from build123d import *

# Parameters (mm, degrees)
F0_W     = 2
F0_H     = 10
F1_DEPTH = 2
F3_D     = 1
F3_DEPTH = 8
F5_D     = 1
F5_DEPTH = 8


with BuildPart() as f1:
    # F0 (on Front) → F1 (new body)
    with BuildSketch(Plane.XZ):
        Rectangle(F0_W, F0_H)
    extrude(amount=F1_DEPTH)

    # F3
    with Locations(Plane.XZ.offset(2)):
        with Locations((0, 4)):
            Hole(F3_D / 2, depth=F3_DEPTH)

    # F5
    with Locations(Plane.YZ.offset(1)):
        with Locations((-1, 2.5)):
            Hole(F5_D / 2, depth=F5_DEPTH)


solid = f1.part
The model under review builds one solid part; all positions refer to its coordinate system, in mm. Round coordinates to 2 decimals unless told otherwise and drop trailing zeros. Loops run counter-clockwise (first coordinate to the right, second up) from the corner with the lowest first, then second, coordinate; pieces in that order, holes last. Notation, with made-up numbers: (-7, -33.75) -> (37, -33.75) arc R17 cw to (37, -3.75) -> close; hole circle Ø5 at (-7.5, -12.75). An arc over 180 degrees is marked (long way). Return JSON: item names as keys, results as strings.
(1) The part is to be moulded in two halves that separate along Y. For faces 1 (the cylindrical face through (0, -1, 3)), 2 (the flat face through (0, -1, -5)), 3 (the flat face through (0, -2, 0)), say which applies: released by +Y, released by -Y, zero draft, split by the parting line, or undercut.
Solved:
{"face 1": "undercut", "face 2": "zero draft", "face 3": "released by -Y"}
(2) Add section C-C on y = -0.9. Write out the cut boundary in (x, z), plus the area to 3 significant figures.
Solved:
{"outline": "(-1, -5) -> (1, -5) -> (1, 2.01) -> (-1, 2.01) -> close; (-1, 2.99) -> (1, 2.99) -> (1, 5) -> (-1, 5) -> close; hole circle Ø1 at (0, 4)", "area": "17.3 mm2"}
(3) For line 1 (Z direction, x = 0, y = -0.8); line 2 (Z direction, x = 0, y = -1.35); line 3 (X direction, y = -0.2, z = 4.25), list the stretches that pass through material, from the lowest coordinate up.
Solved:
{"line 1": "-5 to 2.04, 2.96 to 3.5, 4.5 to 5", "line 2": "-5 to 2.14, 2.86 to 3.5, 4.5 to 5", "line 3": "-1 to -0.43, 0.43 to 1"}
(4) Add section B-B on z = 4. Write out the cut boundary in (x, y), plus the area to 3 significant figures.
Solved:
{"outline": "(-1, -2) -> (-0.5, -2) -> (-0.5, 0) -> (-1, 0) -> close; (0.5, -2) -> (1, -2) -> (1, 0) -> (0.5, 0) -> close", "area": "2.00 mm2"}
(5) Add section D-D on x = -0.6. Write out the cut boundary in (y, z).
Solved:
{"outline": "(-2, -5) -> (0, -5) -> (0, 5) -> (-2, 5) -> close; hole circle Ø1 at (-1, 2.5)"}
(6) Add section A-A on x = 0. Write out the cut boundary in (y, z).
Solved:
{"outline": "(-2, -5) -> (0, -5) -> (0, 3.5) -> (-2, 3.5) -> close; (-2, 4.5) -> (0, 4.5) -> (0, 5) -> (-2, 5) -> close; hole circle Ø1 at (-1, 2.5)"}
